Here's how the part is built. I have some questions about the finished solid (model axes, mm). Face numbers are marked on the shaded views. Give positions to 0.01 mm unless a question says otherwise; leave off trailing zeros. Loops run counter-clockwise (first coordinate to the right, second up) from the corner with the lowest first, then second, coordinate; pieces in that order, holes last. Notation, with made-up numbers: (56, 15) -> (63, 15) arc R14 cw to (63, 33) -> close; hole circle Ø3 at (-10, 42). An arc over 180 degrees is marked (long way). Answer in a Markdown table with one row per item. Add a question column.
Item 1: If we section it at C-C (y = -4.75): Write out the boundary of the cut face in (x, z).
Item 2: We'd pull the mould along Z, two halves only. Please class the marked faces 1, 2 and 3: released by +Z, released by -Z, zero draft, split by the parting line, or undercut.
Item 3: If I drill on line 1 (X direction, y = 7.1, z = 36.05); line 2 (X direction, y = 6.15, z = 26.05); line 3 (X direction, y = 5.5, z = -27.5) (3 decimals), over which ranges is the centre line in solid material (lowest first)?
Item 4: If we section it at A-A (z = 36.05): Write out the boundary of the cut face in (x, y), then the cut area to 3 significant figures.
Item 5: If we section it at B-B (y = 3.25): Write out the boundary of the cut face in (x, z), then the cut area to 3 significant figures.
Item 6: If we section it at D-D (x = 30): Write out the boundary of the cut face in (y, z).
Item 7: For P1, Ø4, axis at x = -37.5, y = -9, coming from the -Z side; P2, Ø2, axis at y = 8.5, z = -22, coming from the -X side; P3, Ø2, axis at y = 9, z = -21.5, coming from the +X side; P4, Ø4, axis at y = -7, z = 52.5, coming from the +X side, each with a flat end and sliding along its axis, tell me the tip position at first contact or that it passes through.
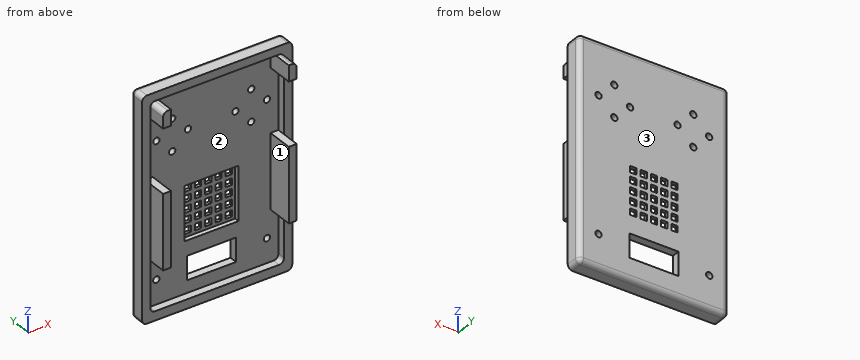
```python
from build123d import *

# Parameters (mm, degrees)
SKETCH1_W           = 95
SKETCH1_H           = 140
BOSS_EXTRUDE1_DEPTH = 10
SKETCH7_W           = 5
SKETCH7_H           = 129
BOSS_EXTRUDE3_DEPTH = 11.5
SKETCH8_R           = 2
SKETCH8_W           = 31
SKETCH8_H           = 15
CUT_EXTRUDE1_DEPTH  = 10
SKETCH14_W          = 34
SKETCH14_H          = 34
CUT_EXTRUDE3_DEPTH  = 8
SKETCH13_W          = 4
SKETCH13_H          = 4
CUT_EXTRUDE4_DEPTH  = 7
SKETCH15_W          = 74.5
SKETCH15_H          = 129
CUT_EXTRUDE5_DEPTH  = 5
CUT_EXTRUDE8_REACH  = 89.284
SKETCH18_W          = 5
SKETCH18_H          = 32
SKETCH18_H_2        = 40
FILLET1_R           = 3


with BuildPart() as part:
    # Sketch1 → Boss-Extrude1 (new body)
    with BuildSketch(Plane(origin=(0, 0, 0), x_dir=(1, 0, 0), z_dir=(0, 1, 0))):
        Rectangle(SKETCH1_W, SKETCH1_H)
    extrude(amount=BOSS_EXTRUDE1_DEPTH)

    # Sketch7 → Boss-Extrude3 (add)
    with BuildSketch(Plane.XZ):
        with Locations((-39.75, 0.25)):
            Rectangle(SKETCH7_W, SKETCH7_H)
        with Locations((39.75, 0.25)):
            Rectangle(SKETCH7_W, SKETCH7_H)
    extrude(amount=BOSS_EXTRUDE3_DEPTH)

    # Sketch8 → Cut-Extrude1 (cut)
    with BuildSketch(Plane(origin=(0, 10, 0), x_dir=(1, 0, 0), z_dir=(0, 1, 0))):
        with Locations(Location((-35, 49, 0), (0, 0, 270))):
            Circle(SKETCH8_R)
        with Locations(Location((35, 49, 0), (0, 0, 270))):
            Circle(SKETCH8_R)
        with Locations(Location((-14.95, -36.05, 0), (0, 0, 270))):
            Circle(SKETCH8_R)
        with Locations(Location((-34.95, -36.05, 0), (0, 0, 270))):
            Circle(SKETCH8_R)
        with Locations(Location((-24.95, -46.05, 0), (0, 0, 270))):
            Circle(SKETCH8_R)
        with Locations(Location((-24.95, -26.05, 0), (0, 0, 270))):
            Circle(SKETCH8_R)
        with Locations(Location((25.05, -26.05, 0), (0, 0, 90))):
            Circle(SKETCH8_R)
        with Locations(Location((35.05, -36.05, 0), (0, 0, 90))):
            Circle(SKETCH8_R)
        with Locations(Location((25.05, -46.05, 0), (0, 0, 90))):
            Circle(SKETCH8_R)
        with Locations(Location((15.05, -36.05, 0), (0, 0, 90))):
            Circle(SKETCH8_R)
        with Locations((-0.05, 48.98)):
            Rectangle(SKETCH8_W, SKETCH8_H)
    extrude(amount=-CUT_EXTRUDE1_DEPTH, mode=Mode.SUBTRACT)

    # Sketch14 → Cut-Extrude3 (cut)
    with BuildSketch(Plane.XZ):
        with Locations((-0.045, -14.99)):
            Rectangle(SKETCH14_W, SKETCH14_H)
    extrude(amount=-CUT_EXTRUDE3_DEPTH, mode=Mode.SUBTRACT)

    # Sketch13 → Cut-Extrude4 (cut)
    with BuildSketch(Plane(origin=(0, 10, 0), x_dir=(1, 0, 0), z_dir=(0, 1, 0))):
        with Locations((-6.545, 27.99)):
            Rectangle(SKETCH13_W, SKETCH13_H)
        with Locations((-13.045, 27.99)):
            Rectangle(SKETCH13_W, SKETCH13_H)
        with Locations((-0.045, 27.99)):
            Rectangle(SKETCH13_W, SKETCH13_H)
        with Locations((6.455, 27.99)):
            Rectangle(SKETCH13_W, SKETCH13_H)
        with Locations((12.955, 27.99)):
            Rectangle(SKETCH13_W, SKETCH13_H)
        with Locations((-6.545, 21.49)):
            Rectangle(SKETCH13_W, SKETCH13_H)
        with Locations((-0.045, 21.49)):
            Rectangle(SKETCH13_W, SKETCH13_H)
        with Locations((6.455, 21.49)):
            Rectangle(SKETCH13_W, SKETCH13_H)
        with Locations((12.955, 21.49)):
            Rectangle(SKETCH13_W, SKETCH13_H)
        with Locations((-6.545, 14.99)):
            Rectangle(SKETCH13_W, SKETCH13_H)
        with Locations((-0.045, 14.99)):
            Rectangle(SKETCH13_W, SKETCH13_H)
        with Locations((6.455, 14.99)):
            Rectangle(SKETCH13_W, SKETCH13_H)
        with Locations((12.955, 14.99)):
            Rectangle(SKETCH13_W, SKETCH13_H)
        with Locations((-6.545, 8.49)):
            Rectangle(SKETCH13_W, SKETCH13_H)
        with Locations((-0.045, 8.49)):
            Rectangle(SKETCH13_W, SKETCH13_H)
        with Locations((6.455, 8.49)):
            Rectangle(SKETCH13_W, SKETCH13_H)
        with Locations((12.955, 8.49)):
            Rectangle(SKETCH13_W, SKETCH13_H)
        with Locations((-6.545, 1.99)):
            Rectangle(SKETCH13_W, SKETCH13_H)
        with Locations((-0.045, 1.99)):
            Rectangle(SKETCH13_W, SKETCH13_H)
        with Locations((6.455, 1.99)):
            Rectangle(SKETCH13_W, SKETCH13_H)
        with Locations((12.955, 1.99)):
            Rectangle(SKETCH13_W, SKETCH13_H)
        with Locations((-13.045, 21.49)):
            Rectangle(SKETCH13_W, SKETCH13_H)
        with Locations((-13.045, 14.99)):
            Rectangle(SKETCH13_W, SKETCH13_H)
        with Locations((-13.045, 8.49)):
            Rectangle(SKETCH13_W, SKETCH13_H)
        with Locations((-13.045, 1.99)):
            Rectangle(SKETCH13_W, SKETCH13_H)
    extrude(amount=-CUT_EXTRUDE4_DEPTH, mode=Mode.SUBTRACT)

    # Sketch15 → Cut-Extrude5 (cut)
    with BuildSketch(Plane.XZ):
        with Locations((0, 0.25)):
            Rectangle(SKETCH15_W, SKETCH15_H)
    extrude(amount=-CUT_EXTRUDE5_DEPTH, mode=Mode.SUBTRACT)

    # Cut-Extrude8: up to this face of the body (flat: up to its plane)
    cut_extrude8_end = Plane(part.part.faces().sort_by_distance((0.008932466, 5, 5.101088901))[0])
    # Sketch18 → Cut-Extrude8 (cut, up to the picked face)
    with BuildSketch(Plane.XZ.offset(11.5), mode=Mode.PRIVATE) as cut_extrude8_sk1:
        with Locations((-39.75, -48.25)):
            Rectangle(SKETCH18_W, SKETCH18_H)
    cut_extrude8_tool1 = split(extrude(cut_extrude8_sk1.sketch, amount=-CUT_EXTRUDE8_REACH, mode=Mode.PRIVATE), bisect_by=cut_extrude8_end, keep=Keep.BOTH, mode=Mode.PRIVATE)
    # Sketch18 → Cut-Extrude8 (cut, up to the picked face)
    with BuildSketch(Plane.XZ.offset(11.5), mode=Mode.PRIVATE) as cut_extrude8_sk2:
        with Locations((-39.75, 34.75)):
            Rectangle(SKETCH18_W, SKETCH18_H_2)
    cut_extrude8_tool2 = split(extrude(cut_extrude8_sk2.sketch, amount=-CUT_EXTRUDE8_REACH, mode=Mode.PRIVATE), bisect_by=cut_extrude8_end, keep=Keep.BOTH, mode=Mode.PRIVATE)
    # Sketch18 → Cut-Extrude8 (cut, up to the picked face)
    with BuildSketch(Plane.XZ.offset(11.5), mode=Mode.PRIVATE) as cut_extrude8_sk3:
        with Locations((39.75, -48.25)):
            Rectangle(SKETCH18_W, SKETCH18_H)
    cut_extrude8_tool3 = split(extrude(cut_extrude8_sk3.sketch, amount=-CUT_EXTRUDE8_REACH, mode=Mode.PRIVATE), bisect_by=cut_extrude8_end, keep=Keep.BOTH, mode=Mode.PRIVATE)
    # Sketch18 → Cut-Extrude8 (cut, up to the picked face)
    with BuildSketch(Plane.XZ.offset(11.5), mode=Mode.PRIVATE) as cut_extrude8_sk4:
        with Locations((39.75, 34.75)):
            Rectangle(SKETCH18_W, SKETCH18_H_2)
    cut_extrude8_tool4 = split(extrude(cut_extrude8_sk4.sketch, amount=-CUT_EXTRUDE8_REACH, mode=Mode.PRIVATE), bisect_by=cut_extrude8_end, keep=Keep.BOTH, mode=Mode.PRIVATE)
    add(cut_extrude8_tool1.solids().sort_by(Axis((-39.75, -11.5, -48.25), (0, 1, 0)))[0], mode=Mode.SUBTRACT)
    add(cut_extrude8_tool2.solids().sort_by(Axis((-39.75, -11.5, 34.75), (0, 1, 0)))[0], mode=Mode.SUBTRACT)
    add(cut_extrude8_tool3.solids().sort_by(Axis((39.75, -11.5, -48.25), (0, 1, 0)))[0], mode=Mode.SUBTRACT)
    add(cut_extrude8_tool4.solids().sort_by(Axis((39.75, -11.5, 34.75), (0, 1, 0)))[0], mode=Mode.SUBTRACT)

    # Fillet1
    fillet1_edges = [part.edges().sort_by_distance(p)[0] for p in [
        (0, 10, -70),
        (47.5, 10, 0),
        (-42.25, -5.75, 64.75),
        (42.25, -5.75, 64.75),
        (0, 10, 70),
        (42.25, 2.5, -64.25),
        (-42.25, 2.5, -64.25),
        (47.5, 5, 70),
        (47.5, 5, -70),
        (-47.5, 5, -70),
        (-47.5, 5, 70),
        (-47.5, 10, 0),
    ]]
    fillet(fillet1_edges, radius=FILLET1_R)


solid = part.part
```
Recorded:
| question | item | result |
|---|---|---|
| 1 | outline | (-42.25, -32.25) -> (-37.25, -32.25) -> (-37.25, 14.75) -> (-42.25, 14.75) -> close; (-42.25, 54.75) -> (-37.25, 54.75) -> (-37.25, 64.75) -> (-39.25, 64.75) arc R3 ccw to (-42.25, 61.75) -> close; (37.25, -32.25) -> (42.25, -32.25) -> (42.25, 14.75) -> (37.25, 14.75) -> close; (37.25, 54.75) -> (42.25, 54.75) -> (42.25, 61.75) arc R3 ccw to (39.25, 64.75) -> (37.25, 64.75) -> close |
| 2 | face 1 | undercut |
| 2 | face 2 | undercut |
| 2 | face 3 | zero draft |
| 3 | line 1 | x = -47.5 to -36.95, -32.95 to -16.95, -12.95 to 13.05, 17.05 to 33.05, 37.05 to 47.5 |
| 3 | line 2 | x = -47.5 to -26.95, -22.95 to 23.05, 27.05 to 47.5 |
| 3 | line 3 | x = -47.5 to -17.045, 16.955 to 47.5 |
| 4 | outline | (-47.5, 0) -> (-42.25, 0) -> (-42.25, 5) -> (-36.95, 5) -> (-36.95, 10) -> (-44.5, 10) arc R3 ccw to (-47.5, 7) -> close; (-32.95, 5) -> (-16.95, 5) -> (-16.95, 10) -> (-32.95, 10) -> close; (-12.95, 5) -> (13.05, 5) -> (13.05, 10) -> (-12.95, 10) -> close; (17.05, 5) -> (33.05, 5) -> (33.05, 10) -> (17.05, 10) -> close; (37.05, 5) -> (42.25, 5) -> (42.25, 0) -> (47.5, 0) -> (47.5, 7) arc R3 ccw to (44.5, 10) -> (37.05, 10) -> close |
| 4 | area | 444 mm^2 |
| 5 | outline | (-47.5, -67) arc R3 ccw to (-44.5, -70) -> (44.5, -70) arc R3 ccw to (47.5, -67) -> (47.5, 67) arc R3 ccw to (44.5, 70) -> (-44.5, 70) arc R3 ccw to (-47.5, 67) -> close; hole (-42.25, -61.25) arc R3 ccw to (-39.25, -64.25) -> (39.25, -64.25) arc R3 ccw to (42.25, -61.25) -> (42.25, -32.25) -> (37.25, -32.25) -> (37.25, 14.75) -> (42.25, 14.75) -> (42.25, 54.75) -> (37.25, 54.75) -> (37.25, 64.75) -> (-37.25, 64.75) -> (-37.25, 54.75) -> (-42.25, 54.75) -> (-42.25, 14.75) -> (-37.25, 14.75) -> (-37.25, -32.25) -> (-42.25, -32.25) -> close |
| 5 | area | 2,970 mm^2 |
| 6 | outline | (0, -70) -> (7, -70) arc R3 ccw to (10, -67) -> (10, 67) arc R3 ccw to (7, 70) -> (0, 70) -> (0, 64.75) -> (5, 64.75) -> (5, -64.25) -> (0, -64.25) -> close |
| 7 | P1 | stops at z = -32.25 |
| 7 | P2 | stops at x = -47.46 |
| 7 | P3 | stops at x = 47.33 |
| 7 | P4 | passes through |
